```python
from build123d import *

# Parameters (mm, degrees)
SKETCH1_R           = 200
BOSS_EXTRUDE1_DEPTH = 2
SKETCH2_R           = 2
CUT_EXTRUDE1_DEPTH  = 13
CIRPATTERN1_COUNT   = 4
SKETCH4_R           = 35
CUT_EXTRUDE3_DEPTH  = 283.849783454


with BuildPart() as part:
    # Sketch1 → Boss-Extrude1 (new body)
    with BuildSketch(Plane.XY):
        Circle(SKETCH1_R)
    extrude(amount=BOSS_EXTRUDE1_DEPTH)

    # Sketch2 → Cut-Extrude1 (cut)
    with BuildSketch(Plane(origin=(0, 0, 0), x_dir=(-1, 0, 0), z_dir=(0, 0, -1))):
        with Locations((11.5, 180)):
            Circle(SKETCH2_R)
        with Locations(Location((-11.5, 180, 0), (0, 0, 180))):
            Circle(SKETCH2_R)
    cut_extrude1 = extrude(amount=-CUT_EXTRUDE1_DEPTH, mode=Mode.SUBTRACT)

    # CirPattern1: Cut-Extrude1 ×4 about axis
    cirpattern1_axis = Axis((0, 0, 0), (0, 0, 1))
    for i in range(1, CIRPATTERN1_COUNT):
        add(cut_extrude1.rotate(cirpattern1_axis, i * 360 / CIRPATTERN1_COUNT), mode=Mode.SUBTRACT)

    # Sketch4 → Cut-Extrude3 (cut, through all)
    with BuildSketch(Plane(origin=(0, 0, 0), x_dir=(-1, 0, 0), z_dir=(0, 0, -1))):
        Circle(SKETCH4_R)
    extrude(amount=-CUT_EXTRUDE3_DEPTH, mode=Mode.SUBTRACT)


solid = part.part
```
Part model, mm, in its own coordinate system. Give positions to 0.01 mm unless a question says otherwise; leave off trailing zeros. Order: outer loops, then holes, each group sorted by start corner. A loop starts at its lowest first (then second) coordinate and runs counter-clockwise, first axis right, second up. Notation, with made-up numbers: (-39, -25.5) - (-3, -25.5) arc R5 ccw to (-3, -16.5) - close; hole circle Ø7 at (-23.5, -1). An arc over 180 degrees is marked (long way). Use one line per item in the form item = value.
Item 1: Slice it at B-B on y = 0. Give the cut face in (x, z).
Solution:
outline = (-200, 0) - (-35, 0) - (-35, 2) - (-200, 2) - close; (35, 0) - (200, 0) - (200, 2) - (35, 2) - close
Item 2: Probe probe 1 along Y at (x, z) = (-11.5, 1.4); probe 2 along Y at (x, z) = (-180, 0.55). List the from-to ranges inside material, lowest first. Write a range as from..to.
Solution:
probe_1 = -199.67..-182, -178..-33.06, 33.06..178, 182..199.67
probe_2 = -87.18..-13.5, -9.5..9.5, 13.5..87.18
Item 3: Slice it at A-A on z = 1.05. Count the separate pieces of the cut face and the enclosed holes in it, and give its area (3 significant figures).
Solution:
separate_pieces = 1
enclosed_holes = 9
area = 122,000 mm2
Item 4: Slice it at D-D on y = -72. Give the cut face in (x, z), and give its area (3 significant figures).
Solution:
outline = (-186.59, 0) - (186.59, 0) - (186.59, 2) - (-186.59, 2) - close
area = 746 mm2
Item 5: Two-plate mould, pull along Y, no slides. Class faces 1 (the face through (190.764, 60.075, 0.986)), 2 (the face through (28, -21, 1)), 3 (the face through (-3, -42, 0)): released by +Y, released by -Y, zero draft, split by the parting line, or undercut.
Solution:
face_1 = split by the parting line
face_2 = undercut
face_3 = zero draft
Item 6: Slice it at C-C on x = -140.5. Give the cut face in (y, z), and give its area (3 significant figures).
Solution:
outline = (-142.34, 0) - (142.34, 0) - (142.34, 2) - (-142.34, 2) - close
area = 569 mm2
Item 7: Pin check, flat tip, straight feed: pin 1 Ø6.5 at (x, y) = (180, 11.5) entering from +Z. Stop position of the tip, or through.
Solution:
pin_1 = 2
